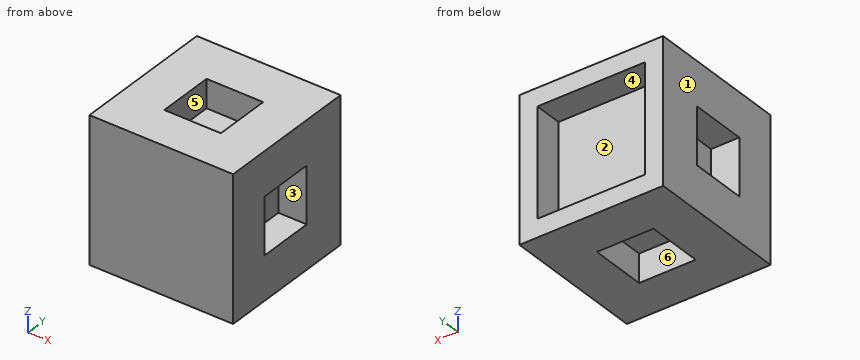
Autodesk Inventor part; units mm, degrees
ref_plane "YZ Plane" through (0, 0, 0) normal (1, 0, 0) x (0, 1, 0)
ref_plane "XZ Plane" through (0, 0, 0) normal (0, 1, 0) x (-1, 0, 0)
ref_plane "XY Plane" through (0, 0, 0) normal (0, 0, 1) x (1, 0, 0)
sketch "Sketch1" plane through (0, 0, 0) normal (0, 1, 0) x (-1, 0, 0)
  line L0 (-12.7, -12.7) -> (-12.7, 12.7)
  line L1 (-12.7, 12.7) -> (12.7, 12.7)
  line L2 (12.7, 12.7) -> (12.7, -12.7)
  line L3 (12.7, -12.7) -> (-12.7, -12.7)
  point P0 (0, 0)
  point P1 (0, 0)
  dimension "d0" = 25.4
extrude "Extrusion1" add sketch "Sketch1" along normal blind 25.4
sketch "Sketch2" plane through (0, 25.4, 0) normal (0, 1, 0) x (1, 0, 0)
  line L0 (9.525, 9.525) -> (9.525, -9.525)
  line L1 (9.525, -9.525) -> (-9.525, -9.525)
  line L2 (-9.525, -9.525) -> (-9.525, 9.525)
  line L3 (-9.525, 9.525) -> (9.525, 9.525)
  point P0 (0, 0)
  point P1 (0, 0)
  dimension "d3" = 19.05
extrude "Extrusion2" cut sketch "Sketch2" against normal blind 5
sketch "Sketch3" plane through (12.7, 0, 12.7) normal (1, 0, 0) x (0, 0, -1)
  line L0 (22.225, 20.4) -> (3.175, 20.4)
  line L1 (17.7, 7.4) -> (7.7, 7.4)
  line L2 (7.7, 7.4) -> (7.7, 17.4)
  line L3 (7.7, 17.4) -> (17.7, 17.4)
  line L4 (17.7, 17.4) -> (17.7, 7.4)
  point P0 (12.7, 0)
  point P1 (12.7, 12.4)
  dimension "d6" = 10
extrude "Extrusion3" cut sketch "Sketch3" against normal blind 5
pattern_circular "Circular Pattern1" count 4 over 360 about axis through (0, -10, 0) along (0, 1, 0) of "Extrusion3"
properties part number "frame_nexus_2"
Design review of the part built by this model. Coordinates are the model's own, in mm. Face numbers are marked on the shaded views. A direction names the side the tool comes from. Round coordinates to 2 decimals unless told otherwise and drop trailing zeros. Write each loop counter-clockwise with the first axis right and the second up, starting at its lowest first coordinate (ties: lowest second). Pieces come first, ordered by that corner, then holes. Notation, with made-up numbers: (22, 85.5) - (32, 85.5) arc R17 cw to (32, 112.5) - close; hole circle Ø7 at (-1, -10). An arc over 180 degrees is marked (long way). Use a Markdown table: item, result. Add a question column.
1. For the marked faces 4, 5 and 6, list the 3-axis set-ups (+Z, -Z, +X, -X, +Y, -Y) from which the entire face can be reached by the end or side of a thin tool; tool diameter is ignored.
2. Mouldability with a two-part tool opening along Y and no side actions: class the marked faces 1, 2 and 3 as +Y half, -Y half, draft (parallel to the pull), parting line (faces both ways), or undercut.
3. We need section D-D (x = -2). State the section outline as (y, z) points (3 decimals).
4. Clearance check with a flat-ended pin moving along its axis: pin 1 (1.5 mm diameter, centred on x = 5, z = -0.5, fed in from +Y). State where the tip first meets the part, or that it passes through.
5. We need section A-A (y = 23.25). State the section outline as (x, z) points (3 decimals), then the cut area to 3 significant figures.
6. We need section B-B (x = -10.25). State the section outline as (y, z) points.
7. We need section C-C (z = 6). State the section outline as (x, y) points (3 decimals).
8. Wall thickness on probe 1 along Z at (x, y) = (4, 24.25) (3 decimals); probe 2 along Y at (x, z) = (-7.75, -3.5); probe 3 along Z at (x, y) = (8.25, 8.75): over which ranges is each line inside the solid? List them lowest first.
Output:
| question | item | result |
|---|---|---|
| 1 | face 4 | +Y |
| 1 | face 5 | +Z |
| 1 | face 6 | -Z |
| 2 | face 1 | draft |
| 2 | face 2 | +Y half |
| 2 | face 3 | undercut |
| 3 | outline | (0, -12.7) - (7.4, -12.7) - (7.4, -7.7) - (17.4, -7.7) - (17.4, -12.7) - (25.4, -12.7) - (25.4, -9.525) - (20.4, -9.525) - (20.4, 9.525) - (25.4, 9.525) - (25.4, 12.7) - (17.4, 12.7) - (17.4, 7.7) - (7.4, 7.7) - (7.4, 12.7) - (0, 12.7) - close |
| 4 | pin 1 | stops at y = 20.4 |
| 5 | outline | (-12.7, -12.7) - (12.7, -12.7) - (12.7, 12.7) - (-12.7, 12.7) - close; hole (-9.525, -9.525) - (9.525, -9.525) - (9.525, 9.525) - (-9.525, 9.525) - close |
| 5 | area | 282 mm2 |
| 6 | outline | (0, -12.7) - (25.4, -12.7) - (25.4, 12.7) - (0, 12.7) - close; hole (7.4, -5) - (17.4, -5) - (17.4, 5) - (7.4, 5) - close |
| 7 | outline | (-12.7, 0) - (12.7, 0) - (12.7, 25.4) - (9.525, 25.4) - (9.525, 20.4) - (-9.525, 20.4) - (-9.525, 25.4) - (-12.7, 25.4) - close |
| 8 | probe 1 | z = -12.7 to -9.525, 9.525 to 12.7 |
| 8 | probe 2 | y = 0 to 7.4, 17.4 to 20.4 |
| 8 | probe 3 | z = -12.7 to -5, 5 to 12.7 |
